from build123d import *

# Parameters (mm, degrees)
CROQUIS1_W              = 150
CROQUIS1_H              = 223
SALIENTE_EXTRUIR1_DEPTH = 100
CROQUIS2_W              = 130
CROQUIS2_H              = 203
SALIENTE_EXTRUIR2_DEPTH = 20
CROQUIS3_R              = 5
CORTAR_EXTRUIR1_DEPTH   = 6


with BuildPart() as part:
    # Croquis1 → Saliente-Extruir1 (new body)
    with BuildSketch(Plane(origin=(0, 0, 0), x_dir=(0, 0, -1), z_dir=(1, 0, 0))):
        Rectangle(CROQUIS1_W, CROQUIS1_H)
    extrude(amount=SALIENTE_EXTRUIR1_DEPTH)

    # Croquis2 → Saliente-Extruir2 (add)
    with BuildSketch(Plane(origin=(100, 0, 0), x_dir=(0, 0, -1), z_dir=(1, 0, 0))):
        Rectangle(CROQUIS2_W, CROQUIS2_H)
    extrude(amount=SALIENTE_EXTRUIR2_DEPTH)

    # Croquis3 → Cortar-Extruir1 (cut)
    with BuildSketch(Plane(origin=(120, 0, 0), x_dir=(0, 0, -1), z_dir=(1, 0, 0))):
        with Locations((-50, -89.5)):
            Circle(CROQUIS3_R)
        with Locations((50, -89.5)):
            Circle(CROQUIS3_R)
    extrude(amount=-CORTAR_EXTRUIR1_DEPTH, mode=Mode.SUBTRACT)


solid = part.part
The listing builds one solid part. Answer for the finished solid, in the listing's coordinates (mm). A direction names the side the tool comes from. Give positions to 0.01 mm unless a question says otherwise; leave off trailing zeros. Loops run counter-clockwise (first coordinate to the right, second up) from the corner with the lowest first, then second, coordinate; pieces in that order, holes last. Notation, with made-up numbers: M 16.5,87.5 L 39.5,87.5 A28 cw 39.5,105.5 Z; hole C 59,19 d11. An arc over 180 degrees is marked long. Answer as CSV lines item,"result".
Item 1: Given pin 1 Ø9 at (y, z) = (-89.5, -50) entering from +X; pin 2 Ø10 at (x, z) = (112, 2) entering from +Y; pin 3 Ø22 at (x, y) = (115, -9) entering from -Z, each flat-ended and moving along its own axis, determine where each tip first touches the part or whether it passes through.
Values follow:
pin 1,"stops at x = 114"
pin 2,"stops at y = 101.5"
pin 3,"stops at z = -65"
Item 2: The mould has two halves that part along Z. Classify faces 1 (the flat face through (100, 9, 67)), 2 (the cylindrical face through (117.04, -94.38, -48.92)), 3 (the flat face through (114, -89, 50)), 4 (the flat face through (110, -1, -65)): released by +Z, released by -Z, zero draft, split by the parting line, or undercut.
Values follow:
face 1,"zero draft"
face 2,"undercut"
face 3,"undercut"
face 4,"released by -Z"
Item 3: The part is cut by section C-C (y = -89.5). Give the vertices of the cut face in (x, z), and give its area (3 significant figures).
Values follow:
outline,"M 0,-75 L 100,-75 L 100,-65 L 120,-65 L 120,-55 L 114,-55 L 114,-45 L 120,-45 L 120,45 L 114,45 L 114,55 L 120,55 L 120,65 L 100,65 L 100,75 L 0,75 Z"
area,"17,500 mm^2"
Item 4: Straight lines are drawn through the part: line 1 along Z through (x, y) = (118, -89); line 2 along Y through (x, z) = (116.75, 50); line 3 along Z through (x, y) = (107, -74). For each, find the intervals that lie inside material, in ascending order. Write a range as [from, to].
Values follow:
line 1,"z = [-65, -54.97], [-45.03, 45.03], [54.97, 65]"
line 2,"y = [-101.5, -94.5], [-84.5, 101.5]"
line 3,"z = [-65, 65]"
Item 5: Which of the six approach directions +Z, -Z, +X, -X, +Y, -Y give full straight-line access (tool end or side, diameter ignored) to faces 5 (the flat face through (110, -101.5, 1)), 6 (the flat face through (110, 101.5, 1)), 7 (the cylindrical face through (117.04, -94.38, 51.08)), 8 (the flat face through (110, -1, 65))?
Values follow:
face 5,"+Z, -Z, +X, -Y"
face 6,"+Z, -Z, +X, +Y"
face 7,"+X"
face 8,"+Z, +X, +Y, -Y"
Item 6: The part is cut by section D-D (z = 52). Give the vertices of the cut face in (x, y).
Values follow:
outline,"M 0,-111.5 L 100,-111.5 L 100,-101.5 L 120,-101.5 L 120,-94.08 L 114,-94.08 L 114,-84.92 L 120,-84.92 L 120,101.5 L 100,101.5 L 100,111.5 L 0,111.5 Z"
Item 7: The part is cut by section A-A (z = -50). Give the vertices of the cut face in (x, y).
Values follow:
outline,"M 0,-111.5 L 100,-111.5 L 100,-101.5 L 120,-101.5 L 120,-94.5 L 114,-94.5 L 114,-84.5 L 120,-84.5 L 120,101.5 L 100,101.5 L 100,111.5 L 0,111.5 Z"
Item 8: The part is cut by section B-B (y = 6). Give the vertices of the cut face in (x, z).
Values follow:
outline,"M 0,-75 L 100,-75 L 100,-65 L 120,-65 L 120,65 L 100,65 L 100,75 L 0,75 Z"
